```python
from build123d import *

# Parameters (mm, degrees)
SKETCH_1_W      = 34
SKETCH_1_H      = 50
EXTRUDE_1_DEPTH = 5
SKETCH_2_R      = 2
EXTRUDE_2_DEPTH = 20
SKETCH_3_W      = 34
SKETCH_3_H      = 50
EXTRUDE_3_DEPTH = 5
SKETCH_4_W      = 20
SKETCH_4_H      = 3
EXTRUDE_4_DEPTH = 30
SKETCH_5_R      = 2
EXTRUDE_5_DEPTH = 25


with BuildPart() as part:
    # 草图1 → 凸台-拉伸1 (new body)
    with BuildSketch(Plane.XY):
        with Locations((-4.949270059, 16.999651533)):
            Rectangle(SKETCH_1_W, SKETCH_1_H)
    extrude(amount=EXTRUDE_1_DEPTH)

    # 草图2 → 凸台-拉伸2 (add)
    with BuildSketch(Plane.XY.offset(5)):
        with Locations((-19.949270059, 31.999651533)):
            Circle(SKETCH_2_R)
        with Locations((-19.949270059, 1.999651533)):
            Circle(SKETCH_2_R)
        with Locations((10.050729941, 31.999651533)):
            Circle(SKETCH_2_R)
        with Locations((10.050729941, 1.999651533)):
            Circle(SKETCH_2_R)
    extrude(amount=EXTRUDE_2_DEPTH)

    # 草图3 → 凸台-拉伸3 (add)
    with BuildSketch(Plane.XY.offset(25)):
        with Locations((-4.949270059, 17.194555641)):
            Rectangle(SKETCH_3_W, SKETCH_3_H)
    extrude(amount=EXTRUDE_3_DEPTH)

    # 草图4 → 凸台-拉伸4 (add)
    with BuildSketch(Plane.XY.offset(30)):
        with Locations((-4.949270059, 30.694555641)):
            Rectangle(SKETCH_4_W, SKETCH_4_H)
        with Locations((-4.949270059, 3.694555641)):
            Rectangle(SKETCH_4_W, SKETCH_4_H)
    extrude(amount=EXTRUDE_4_DEPTH)

    # 草图5 → 凸台-拉伸5 (add)
    with BuildSketch(Plane(origin=(0, 5.194555641, 0), x_dir=(1, 0, 0), z_dir=(0, 1, 0))):
        with Locations((-4.949270059, -45)):
            Circle(SKETCH_5_R)
    extrude(amount=EXTRUDE_5_DEPTH)


solid = part.part
```
Here's how the part is built. I have some questions about the finished solid (model axes, mm). A direction names the side the tool comes from. Give positions to 0.01 mm unless a question says otherwise; leave off trailing zeros. Write each loop counter-clockwise with the first axis right and the second up, starting at its lowest first coordinate (ties: lowest second). Pieces come first, ordered by that corner, then holes. Notation, with made-up numbers: M 32,87 L 85,87 A14 ccw 85,114 Z; hole C -4.5,38 d5. An arc over 180 degrees is marked long. Put each result on its own line as item: value. Start each with the question number.
Item 1: Thinking about a two-plate mould opening in Y: for faces 6 (the cylindrical face through (10, 30, 15)), 7 (the flat face through (-5, 32.195, 45)), 8 (the flat face through (-5, 31, 60)), 9 (the flat face through (-5, 2.195, 45)), which applies, +Y half, -Y half, draft (parallel to the pull), parting line (faces both ways), or undercut?
Item 2: On a 3-axis mill with a long thin cutter (end or side, diameter ignored), from which of +Z, -Z, +X, -X, +Y, -Y can I reach the whole of each face in a straight line? I mean faces 1 (the flat face through (-21.949, 17, 27)), 2 (the flat face through (-14.949, 4, 45)), 3 (the flat face through (5.051, 4, 45)), 4 (the cylindrical face through (-18.04, 2.6, 14.86)), 5 (the flat face through (-5, -7.805, 27)). Say none if no direction works.
Item 3: If we section it at A-A, the plane y = 15: Write out the boundary of the cut face in (x, z).
Item 4: If we section it at C-C, the plane x = 0.5: Write out the boundary of the cut face in (y, z), then the cut area to 3 significant figures.
Item 5: I need wall thicknesses on L1, parallel to Z at x = -14, y = 7; L2, parallel to Y at x = -0.5, z = 38.5; L3, parallel to Y at x = -1.5, z = 29. Which ranges of each line are inside material? Lowest first, please. Write a range as from..to.
Item 6: Will these pins go through, and if not, where does the flat tip stop? pin 1 (3.5 mm diameter, centred on y = 4.5, z = 47.5, fed in from +X); pin 2 (8 mm diameter, centred on y = 26, z = 39, fed in from -X); pin 3 (2.5 mm diameter, centred on x = -1.5, z = 28, fed in from -Y).
Item 7: If we section it at B-B, the plane z = 34: Write out the boundary of the cut face in (x, y), then the cut area to 3 significant figures.
Item 8: If we section it at D-D, the plane x = -6: Write out the boundary of the cut face in (y, z).
Values:
1. face 6: undercut
1. face 7: +Y half
1. face 8: draft
1. face 9: -Y half
2. face 1: +Z, -Z, -X, +Y, -Y
2. face 2: +Z, -X, +Y, -Y
2. face 3: +Z, +X, +Y, -Y
2. face 4: none
2. face 5: +Z, +X, -X, -Y
3. outline: M -21.95,0 L 12.05,0 L 12.05,5 L -21.95,5 Z; M -21.95,25 L 12.05,25 L 12.05,30 L -21.95,30 Z; C -4.95,45 d4
4. outline: M -8,0 L 42,0 L 42,5 L -8,5 Z; M -7.81,25 L 42.19,25 L 42.19,30 L 32.19,30 L 32.19,60 L 29.19,60 L 29.19,30 L 5.19,30 L 5.19,60 L 2.19,60 L 2.19,30 L -7.81,30 Z
4. area: 680 mm²
5. L1: 0..5, 25..30
5. L2: 2.19..5.19, 29.19..32.19
5. L3: -7.81..42.19
6. pin 1: x = 5.05
6. pin 2: x = -14.95
6. pin 3: y = -7.81
7. outline: M -14.95,2.19 L 5.05,2.19 L 5.05,5.19 L -14.95,5.19 Z; M -14.95,29.19 L 5.05,29.19 L 5.05,32.19 L -14.95,32.19 Z
7. area: 120 mm²
8. outline: M -8,0 L 42,0 L 42,5 L -8,5 Z; M -7.81,25 L 42.19,25 L 42.19,30 L 32.19,30 L 32.19,60 L 29.19,60 L 29.19,46.7 L 5.19,46.7 L 5.19,60 L 2.19,60 L 2.19,30 L -7.81,30 Z; hole M 5.19,30 L 29.19,30 L 29.19,43.3 L 5.19,43.3 Z
